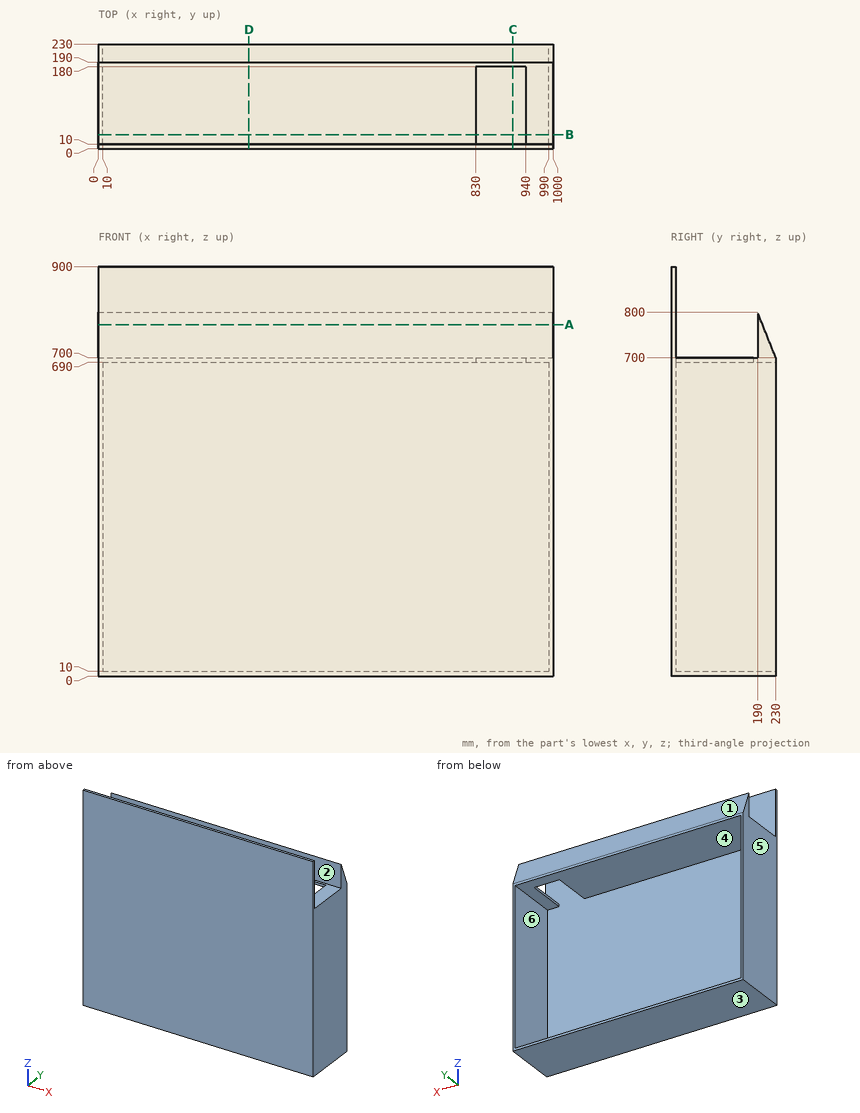
Print and shaded views of the part. All mm, measured from the part's lowest x, y and z. A direction names the side the tool comes from. Give positions to 0.01 mm unless a question says otherwise; leave off trailing zeros. Write each loop counter-clockwise with the first axis right and the second up, starting at its lowest first coordinate (ties: lowest second). Pieces come first, ordered by that corner, then holes. Notation, with made-up numbers: (-17, 81.5) - (8, 81.5) arc R25 cw to (8, 119.5) - close; hole circle Ø8 at (-19.75, 49.5). An arc over 180 degrees is marked (long way). Put each result on its own line as item: value.
(1) Saw through at A-A (z = 772.5). List the corners of the cut face in (x, y).
Working result:
outline: (0, 0) - (1000, 0) - (1000, 10) - (0, 10) - close; (0, 190) - (1000, 190) - (1000, 201) - (0, 201) - close
(2) Saw through at C-C (x = 911.5). List the corners of the cut face in (y, z).
Working result:
outline: (0, 0) - (230, 0) - (230, 10) - (10, 10) - (10, 900) - (0, 900) - close; (180, 690) - (230, 690) - (230, 700) - (190, 800) - (190, 700) - (180, 700) - close
(3) Wall check: L1, parallel to X at y = 185, z = 370; L2, parallel to Z at x = 219.5, y = 95.5; L3, parallel to Y at x = 120, z = 144.5. Give the ranges that are in metal, low to high.
Working result:
L1: 0 to 10, 990 to 1000
L2: 0 to 10, 690 to 700
L3: 0 to 10
(4) Tool access for the marked faces 1 and 2: list every direction of +Z, -Z, +X, -X, +Y, -Y with a clear straight run to the whole face (end or side of a thin tool).
Working result:
face 1: +Z, +X, -X, +Y
face 2: +Z, +X, -X
(5) Saw through at D-D (x = 331). List the corners of the cut face in (y, z).
Working result:
outline: (0, 0) - (230, 0) - (230, 10) - (10, 10) - (10, 690) - (230, 690) - (230, 700) - (190, 800) - (190, 700) - (10, 700) - (10, 900) - (0, 900) - close
(6) Saw through at B-B (y = 30.5). List the corners of the cut face in (x, z).
Working result:
outline: (0, 0) - (1000, 0) - (1000, 700) - (940, 700) - (940, 690) - (990, 690) - (990, 10) - (10, 10) - (10, 690) - (830, 690) - (830, 700) - (0, 700) - close
(7) Drop flat-ended pins along their axis: pin 1 Ø2 at (x, y) = (538.5, 145.5) entering from +Z; pin 2 Ø10 at (x, z) = (820, 245) entering from +Y. Give the stop position or say it passes through.
Working result:
pin 1: z = 700
pin 2: y = 10
(8) Pull direction X, two halves, no side cores. Call the marked faces 3, 4, 5 and 6: released by +X, released by -X, zero draft, split by the parting line, or undercut.
Working result:
face 3: zero draft
face 4: undercut
face 5: released by -X
face 6: undercut
